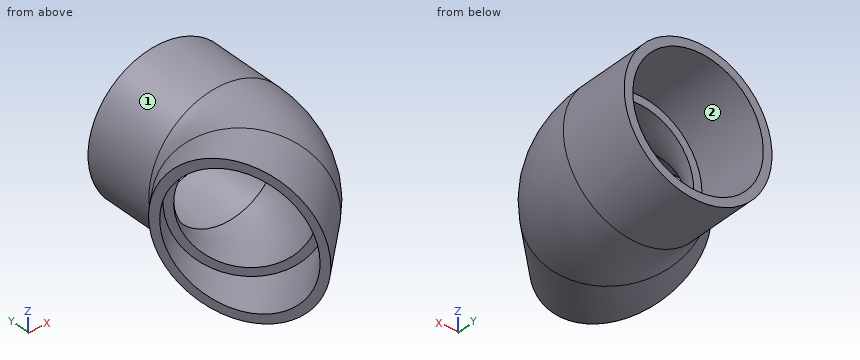
from build123d import *

# Parameters (mm, degrees)
SKETCH3_R               = 34.3535
SKETCH3_R_2             = 26.2509
CUT_EXTRUDE1_DEPTH      = 92.704245656
CUT_EXTRUDE1_DEPTH_BACK = 92.704245656


with BuildPart() as part:
    # Sketch1 → Revolve1 (revolve)
    with BuildSketch(Plane.XY):
        Polygon((-11.539629116, -60.122814731), (13.066272656, -35.516912959), (10.048906599, -32.499546902), (-14.395350562, -57.267093284), align=None)
    revolve(axis=Axis((-35.831221923, -35.831221923, 0), (0.7071067811865488, 0.7071067811865464, 0)))



with BuildPart() as body_2:
    # Sketch2 → Revolve2 (revolve)
    with BuildSketch(Plane.XY, mode=Mode.PRIVATE) as revolve2_sk:
        Polygon((30.3149, 50.673), (30.0863, 15.875), (34.3535, 15.875), (34.3535, 50.673), align=None)
    revolve(revolve2_sk.sketch.rotate(Axis((0, 0, 0), (0, 1, 0)), 90), axis=Axis((0, 0, 0), (0, 1, 0)))


with BuildPart() as part_1:
    add(part.part)

    add(body_2.part)  # Sweep1 merges body 2
    # Sweep1: sweep along a path in Sketch4
    with BuildLine(Plane.XY) as sweep1_path:
        ThreePointArc((-11.225320151, -11.225320151), (-2.917365657, 1.208412421), (0, 15.875))
    # Sketch3 → Sweep1 (sweep)
    with BuildSketch(Plane(origin=(-11.225320151, -11.225320151, 0), x_dir=(0, 0, -1), z_dir=(0.7071067811865486, 0.7071067811865465, 0))):
        Circle(SKETCH3_R)
        Circle(SKETCH3_R_2, mode=Mode.SUBTRACT)
    sweep(path=sweep1_path.line)

    # Sketch5 → Cut-Extrude1 (cut, two sides: drawn at the far end of the back side and taken through both)
    with BuildSketch(Plane.XY.offset(-CUT_EXTRUDE1_DEPTH_BACK)):
        Polygon((-42.162302488, 6.420883127), (-60.122814731, -11.539629116), (-11.539629116, -60.122814731), align=None)
    extrude(amount=CUT_EXTRUDE1_DEPTH + CUT_EXTRUDE1_DEPTH_BACK, mode=Mode.SUBTRACT)


solid = part_1.part
For this review, take the finished solid that the model builds, in its own axes (mm). Face numbers are marked on the shaded views. Give positions to 0.01 mm unless a question says otherwise; leave off trailing zeros. Loops run counter-clockwise (first coordinate to the right, second up) from the corner with the lowest first, then second, coordinate; pieces in that order, holes last.
Item 1: Take a section at A-A, the plane y = 21. State the section outline as (x, z) points.
Item 2: For line 1 along X through (y, z) = (34.5, -2); line 2 along X through (y, z) = (0, 12.5); line 3 along Z through (x, y) = (-11.5, -33.5), list the stretches that pass through material, from the lowest coordinate up.
Item 3: Draft analysis for pull direction X (two halves, no side actions). For the marked faces 1 and 2, state which applies: +X half, -X half, draft (parallel to the pull), parting line (faces both ways), or undercut.
Item 4: Insertion check: pin 1 (1.5 mm diameter, centred on y = -38, z = -20, fed in from -X); pin 2 (12 mm diameter, centred on y = -2.5, z = -6.5, fed in from +X); pin 3 (8 mm diameter, centred on y = 22.5, z = 13, fed in from +X). Each pin has a flat end and moves straight along its axis. Give the tip position at first contact, or say it passes through.
Calculated:
1. outline: circle Ø68.71 at (0, 0); hole circle Ø60.24 at (0, 0)
2. line 1: x = -34.3 to -30.14, 30.14 to 34.3
2. line 2: x = -39.21 to -38.82, 21 to 30.18
2. line 3: z = -30.63 to -25.87, 25.87 to 30.63
3. face 1: parting line
3. face 2: undercut
4. pin 1: stops at x = -7.23
4. pin 2: stops at x = 32.97
4. pin 3: stops at x = 33.15
